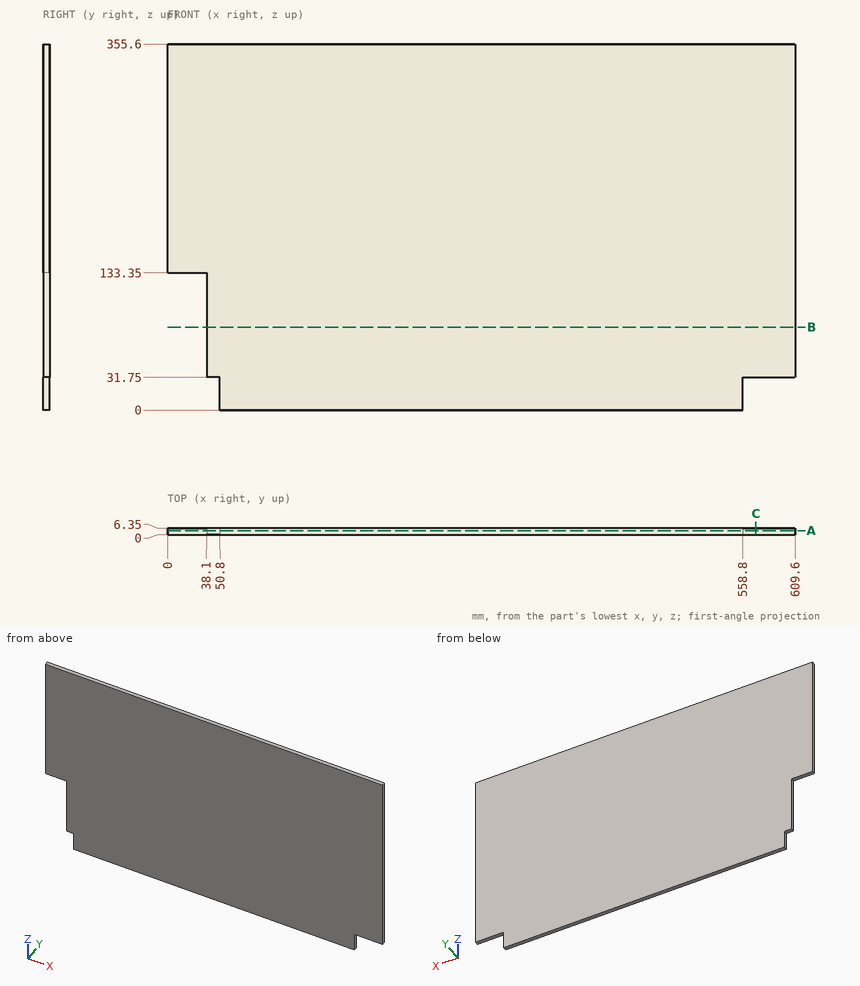
Study the drawing (mm; zero at the part's minimum x, y, z) and answer. Give positions to 0.01 mm unless a question says otherwise; leave off trailing zeros. Write each loop counter-clockwise with the first axis right and the second up, starting at its lowest first coordinate (ties: lowest second). Pieces come first, ordered by that corner, then holes. Notation, with made-up numbers: (64, -11.75) - (113, -11.75) arc R16 ccw to (113, 8.25) - close; hole circle Ø4 at (88.25, 43.5). An arc over 180 degrees is marked (long way). One line per question, with ' | ' between items. Start each with the question number.
1. Section B-B, the plane z = 80.5 is taken. Determine the outline of the cut face in (x, y), then the cut area to 3 significant figures.
2. Section A-A, the plane y = 3.75 is taken. Determine the outline of the cut face in (x, z), then the cut area to 3 significant figures.
3. Section C-C, the plane x = 571.5 is taken. Determine the outline of the cut face in (y, z), then the cut area to 3 significant figures.
4. Straight lines are drawn through the part: line 1 (X direction, y = 5.5, z = 116); line 2 (Z direction, x = 39.5, y = 4); line 3 (X direction, y = 3.5, z = 20). For each, find the intervals that lie inside material, in ascending order.
5. Given P1, Ø1.9, axis at x = 44.5, y = 2, coming from the -Z side; P2, Ø1.9, axis at y = 3.5, z = 23.5, coming from the +X side, each flat-ended and moving along its own axis, determine where each tip first touches the part or whether it passes through.
Result:
1) outline: (38.1, 0) - (609.6, 0) - (609.6, 6.35) - (38.1, 6.35) - close | area: 3,630 mm2
2) outline: (0, 133.35) - (38.1, 133.35) - (38.1, 31.75) - (50.8, 31.75) - (50.8, 0) - (558.8, 0) - (558.8, 31.75) - (609.6, 31.75) - (609.6, 355.6) - (0, 355.6) - close | area: 210,000 mm2
3) outline: (0, 31.75) - (6.35, 31.75) - (6.35, 355.6) - (0, 355.6) - close | area: 2,060 mm2
4) line 1: x = 38.1 to 609.6 | line 2: z = 31.75 to 355.6 | line 3: x = 50.8 to 558.8
5) P1: stops at z = 31.75 | P2: stops at x = 558.8
